Model file for the job. Use its own axes, mm. A direction names the side the tool comes from. Coordinates: 2 decimals unless noted, no trailing zeros. Write each loop counter-clockwise with the first axis right and the second up, starting at its lowest first coordinate (ties: lowest second). Pieces come first, ordered by that corner, then holes. Notation, with made-up numbers: (82.5, 6.25) -> (128.5, 6.25) arc R32 ccw to (128.5, 39.25) -> close; hole circle Ø7 at (16, -27). An arc over 180 degrees is marked (long way). Answer as a JSON object with one key per item and string values. Group by question number.
from build123d import *

# Parameters (mm, degrees)
F0_W     = 10
F0_H     = 10
F1_DEPTH = 12


# Not quite as in the source:
# - ends of sketch curves that miss each other by under 0.0002 mm in the source are joined


with BuildPart() as f1:
    # F0 (on Top) → F1 (new body)
    with BuildSketch(Plane.XY):
        with BuildLine():
            ThreePointArc((49.3437788486, 31.9918581452), (44.6574873088, 43.3055665732), (33.3437788486, 47.9918580353))
            ThreePointArc((33.3437788486, 47.9918580353), (24.3995068895, 45.2583572735), (18.51138183, 37.9918580353))
            Line((18.51138183, 37.9918580353), (33.3437788486, 37.9918580353))
            ThreePointArc((33.3437788486, 37.9918580353), (37.5864194969, 36.2344987613), (39.3437788486, 31.9918581452))
            Line((39.3437788486, 31.9918581452), (39.3437788486, 17.1594610611))
            ThreePointArc((39.3437788486, 17.1594610611), (46.6102780408, 23.0475861709), (49.3437788486, 31.9918581452))
        make_face()
        with BuildLine():
            Line((49.3437788486, -68.0081418548), (49.3437788486, 31.9918581452))
            ThreePointArc((49.3437788486, 31.9918581452), (46.6102780408, 23.0475861709), (39.3437788486, 17.1594610611))
            Line((39.3437788486, 17.1594610611), (39.3437788486, -68.0081418548))
            ThreePointArc((39.3437788486, -68.0081418548), (33.3437788486, -74.0081418548), (27.3437788486, -68.0081418548))
            Line((27.3437788486, -68.0081418548), (27.3437788486, 15.9918580353))
            Line((27.3437788486, 15.9918580353), (17.3437788486, 15.9918580353))
            Line((17.3437788486, 15.9918580353), (17.3437788486, -68.0081418548))
            ThreePointArc((17.3437788486, -68.0081418548), (33.3437788486, -84.0081418548), (49.3437788486, -68.0081418548))
        make_face()
        with BuildLine():
            Line((33.3437788486, 37.9918580353), (18.51138183, 37.9918580353))
            ThreePointArc((18.51138183, 37.9918580353), (17.6383919973, 35.0481342863), (17.3437788486, 31.9918581452))
            Line((17.3437788486, 31.9918581452), (17.3437788486, 25.9918580353))
            Line((17.3437788486, 25.9918580353), (27.3437788486, 25.9918580353))
            Line((27.3437788486, 25.9918580353), (27.3437788486, 31.9918581452))
            ThreePointArc((27.3437788486, 31.9918581452), (29.1011381615, 36.2344988323), (33.3437788486, 37.9918580353))
        make_face()
        with Locations((22.3437788486, 20.9918580353)):
            Rectangle(F0_W, F0_H)
        with BuildLine():
            Line((33.3437788486, 47.9918580353), (-46.6562211514, 47.9918580353))
            ThreePointArc((-46.6562211514, 47.9918580353), (-62.6562211514, 31.9918580353), (-46.6562211514, 15.9918580353))
            Line((-46.6562211514, 15.9918580353), (17.3437788486, 15.9918580353))
            Line((17.3437788486, 15.9918580353), (17.3437788486, 25.9918580353))
            Line((17.3437788486, 25.9918580353), (-46.6562211514, 25.9918580353))
            ThreePointArc((-46.6562211514, 25.9918580353), (-52.6562211514, 31.9918580353), (-46.6562211514, 37.9918580353))
            Line((-46.6562211514, 37.9918580353), (18.51138183, 37.9918580353))
            ThreePointArc((18.51138183, 37.9918580353), (24.3995068895, 45.2583572735), (33.3437788486, 47.9918580353))
        make_face()
    extrude(amount=F1_DEPTH)


solid = f1.part
(1) Pull direction Y, two halves, no side cores. Call faces 1 (the face through (33, -74, 6)), 2 (the face through (-15, 15.992, 6)), 3 (the face through (17.344, 29, 6)), 4 (the face through (18, 2, 0)): released by +Y, released by -Y, zero draft, split by the parting line, or undercut.
(2) Wall check: probe 1 along X at (y, z) = (32, 10); probe 2 along X at (y, z) = (-3.5, 11.5); probe 3 along Y at (x, z) = (17, 5). Give the ranges that are in metal, low to high.
(3) Cut at C-C on z = 10. List the corners of the cut face in (x, y).
(4) Pin check, flat tips, straight feed: pin 1 (1.5 mm diameter, centred on x = -2.5, z = 3, fed in from -Y); pin 2 (6 mm diameter, centred on y = 4, z = 5, fed in from -X); pin 3 (3 mm diameter, centred on y = 28, z = 7, fed in from -X). Stop position of each tip, or through.
(5) 3-axis set-ups, long thin cutter, end or side, ignore diameter. For faces 5 (the face through (32.992, -84.004, 5.916)), 6 (the face through (17.344, -25, 6)), 7 (the face through (39.344, -17, 6)): which of +Z, -Z, +X, -X, +Y, -Y reach the whole face in a straight line?
(6) Cut at B-B on y = -65. List the corners of the cut face in (x, z), plus the area to 3 significant figures.
(7) Cut at A-A on x = -44.5. List the corners of the cut face in (y, z).
Results found:
{
 "1": {"face 1": "undercut", "face 2": "released by -Y", "face 3": "undercut", "face 4": "zero draft"},
 "2": {"probe 1": "x = -62.66 to -52.66, 17.34 to 27.34, 39.34 to 49.34", "probe 2": "x = 17.34 to 27.34, 39.34 to 49.34", "probe 3": "y = 15.99 to 25.99, 37.99 to 47.99"},
 "3": {"outline": "(-46.66, 15.99) -> (17.34, 15.99) -> (17.34, -68.01) arc R16 ccw to (49.34, -68.01) -> (49.34, 31.99) arc R16 ccw to (33.34, 47.99) -> (-46.66, 47.99) arc R16 ccw to start; hole (-46.66, 25.99) -> (17.34, 25.99) -> (17.34, 31.99) arc R16 cw to (18.51, 37.99) -> (-46.66, 37.99) arc R6 ccw to start; hole (27.34, -68.01) arc R6 ccw to (39.34, -68.01) -> (39.34, 31.99) arc R6 ccw to (27.34, 31.99) -> close"},
 "4": {"pin 1": "stops at y = 15.99", "pin 2": "stops at x = 17.34", "pin 3": "stops at x = -62.46"},
 "5": {"face 5": "+Z, -Z, -Y", "face 6": "+Z, -Z, -X, -Y", "face 7": "+Z, -Z"},
 "6": {"outline": "(17.34, 0) -> (27.34, 0) -> (27.34, 12) -> (17.34, 12) -> close; (39.34, 0) -> (49.34, 0) -> (49.34, 12) -> (39.34, 12) -> close", "area": "240 mm²"},
 "7": {"outline": "(15.99, 0) -> (25.99, 0) -> (25.99, 12) -> (15.99, 12) -> close; (37.99, 0) -> (47.99, 0) -> (47.99, 12) -> (37.99, 12) -> close"}
}
